CAD build for the part. Positions are in the model's coordinates, mm. Coordinates: 2 decimals unless noted, no trailing zeros. Write each loop counter-clockwise with the first axis right and the second up, starting at its lowest first coordinate (ties: lowest second). Pieces come first, ordered by that corner, then holes.
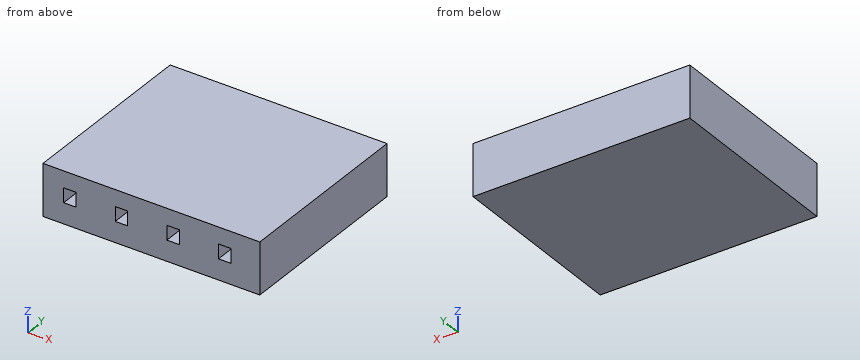
```python
from build123d import *

# Parameters (mm, degrees)
BOX297_W         = 0.6
BOX297_H         = 0.7
BOX297_DEPTH     = 5
ARRAY009_X_COUNT = 4
ARRAY009_X_PITCH = 2.5
BOX296_W         = 2.5
BOX296_H         = 9
BOX296_DEPTH     = 10.5


with BuildPart() as array009:
    # Box297 → Box297 (new body)
    with BuildSketch(Plane(origin=(-27, -22.5, 13.5), x_dir=(1, 0, 0), z_dir=(0, -1, 0))):
        with Locations((0.3, 0.35)):
            Rectangle(BOX297_W, BOX297_H)
    extrude(amount=BOX297_DEPTH)

    # Array009 X: Array009 ×4


with BuildPart() as array009_1:
    add(array009.part)
    with Locations(*[(i * ARRAY009_X_PITCH, 0, 0) for i in range(1, ARRAY009_X_COUNT)]):
        add(array009.part)


with BuildPart() as obj1:
    # Box296 → Box296 (new body)
    with BuildSketch(Plane(origin=(-28, -27, 15), x_dir=(0, 0, -1), z_dir=(1, 0, 0))):
        with Locations((1.25, 4.5)):
            Rectangle(BOX296_W, BOX296_H)
    extrude(amount=BOX296_DEPTH)

    # Cut345: cut Array009
    add(array009_1.part, mode=Mode.SUBTRACT)


solid = obj1.part
```
Item 1: Saw through at A-A, the plane z = 13.75. Write the cut outline in (x, y), and give its area (3 significant figures).
Item 2: Saw through at B-B, the plane y = -24. Write the cut outline in (x, z), and give its area (3 significant figures).
Item 3: Wall check: line 1 along X through (y, z) = (-24.5, 14.1); line 2 along Z through (x, y) = (-26.5, -25.5). Give the ranges that are in metal, low to high.
Working result:
1. outline: (-28, -27) - (-27, -27) - (-27, -22.5) - (-26.4, -22.5) - (-26.4, -27) - (-24.5, -27) - (-24.5, -22.5) - (-23.9, -22.5) - (-23.9, -27) - (-22, -27) - (-22, -22.5) - (-21.4, -22.5) - (-21.4, -27) - (-19.5, -27) - (-19.5, -22.5) - (-18.9, -22.5) - (-18.9, -27) - (-17.5, -27) - (-17.5, -18) - (-28, -18) - close
1. area: 83.7 mm2
2. outline: (-28, 12.5) - (-17.5, 12.5) - (-17.5, 15) - (-28, 15) - close; hole (-27, 13.5) - (-26.4, 13.5) - (-26.4, 14.2) - (-27, 14.2) - close; hole (-24.5, 13.5) - (-23.9, 13.5) - (-23.9, 14.2) - (-24.5, 14.2) - close; hole (-22, 13.5) - (-21.4, 13.5) - (-21.4, 14.2) - (-22, 14.2) - close; hole (-19.5, 13.5) - (-18.9, 13.5) - (-18.9, 14.2) - (-19.5, 14.2) - close
2. area: 24.6 mm2
3. line 1: x = -28 to -27, -26.4 to -24.5, -23.9 to -22, -21.4 to -19.5, -18.9 to -17.5
3. line 2: z = 12.5 to 13.5, 14.2 to 15
